Can you work these out from the model? Positions are in its coordinate system, mm. A direction names the side the tool comes from. Give positions to 0.01 mm unless a question says otherwise; leave off trailing zeros. Order: outer loops, then holes, each group sorted by start corner. A loop starts at its lowest first (then second) coordinate and runs counter-clockwise, first axis right, second up. Notation, with made-up numbers: M 21,6 L 45,6 A17 cw 45,29 Z; hole C 79,-19.5 d5. An arc over 180 degrees is marked long. Write each question's results on one line, items separated by ' | '.
Solid Edge part; units mm, degrees
sketch "Sketch1" plane through (0, 0, 0) normal (0, 0, 1) x (1, 0, 0)
  circle A0 centre (0, 0) radius 17
  circle A1 centre (0, 0) radius 12.25
extrude "Protrusion1" add sketch "Sketch1" along normal blind 20
sketch "Sketch2" plane through (0, 0, 20) normal (0, 0, 1) x (0, 1, 0)
  circle A0 centre (0, 0) radius 12.25
  circle A1 centre (0, 0) radius 14
extrude "Extrusionsausprägung_2" add sketch "Sketch2" along normal blind 5
chamfer "Fase_1" distance 1 angle 45 1 edges at (0, -14, 25)
sketch "Sketch3" plane through (0, 0, 0) normal (0, 0, -1) x (0, 1, 0)
  circle A0 centre (0, 0) radius 14.15
extrude "Extrusionsausschnitt_1" cut sketch "Sketch3" against normal blind 6
(1) I need wall thicknesses on L1, parallel to Y at x = 0, z = 17.25; L2, parallel to X at y = 0.5, z = 3.25; L3, parallel to Z at x = 15, y = 0.5. Which ranges of each line are inside material? Lowest first, please. Write a range as from..to.
Data:
L1: y = -17..-12.25, 12.25..17 | L2: x = -16.99..-14.14, 14.14..16.99 | L3: z = 0..20
(2) For faces 5 (the face through (-6, 13, 20)), 6 (the face through (9.139, -14.334, 9.86)), which set-ups out of +Z, -Z, +X, -X, +Y, -Y let a thin tool reach every point of the face, with its end or its side?
Data:
face 5: +Z | face 6: +Z, -Z
(3) Imagine slicing it at B-B, the plane x = 15.5. Write out the boundary of the cut face in (y, z).
Data:
outline: M -6.98,0 L 6.98,0 L 6.98,20 L -6.98,20 Z
(4) We'd pull the mould along X, two halves only. Please class faces 1 (the face through (-5.362, 12.932, 21.972)), 2 (the face through (-4, 12, 25)), 3 (the face through (4, 12, 6)), 4 (the face through (-12.553, 6.529, 2.958)): +X half, -X half, draft (parallel to the pull), parting line (faces both ways), or undercut.
Data:
face 1: parting line | face 2: draft | face 3: undercut | face 4: undercut
(5) Imagine slicing it at A-A, the plane z = 18.25. Write out the boundary of the cut face in (x, y).
Data:
outline: C 0,0 d34; hole C 0,0 d24.5
(6) Will these pins go through, and if not, where does the flat tip stop? P1, Ø2, axis at y = -7.5, z = 7.5, coming from the +X side; P2, Ø3, axis at y = 11.5, z = 11, coming from the +X side; P3, Ø6, axis at x = 10.5, z = 19.5, coming from the +Y side.
Data:
P1: stops at x = 15.71 | P2: stops at x = 13.75 | P3: stops at y = 15.26
